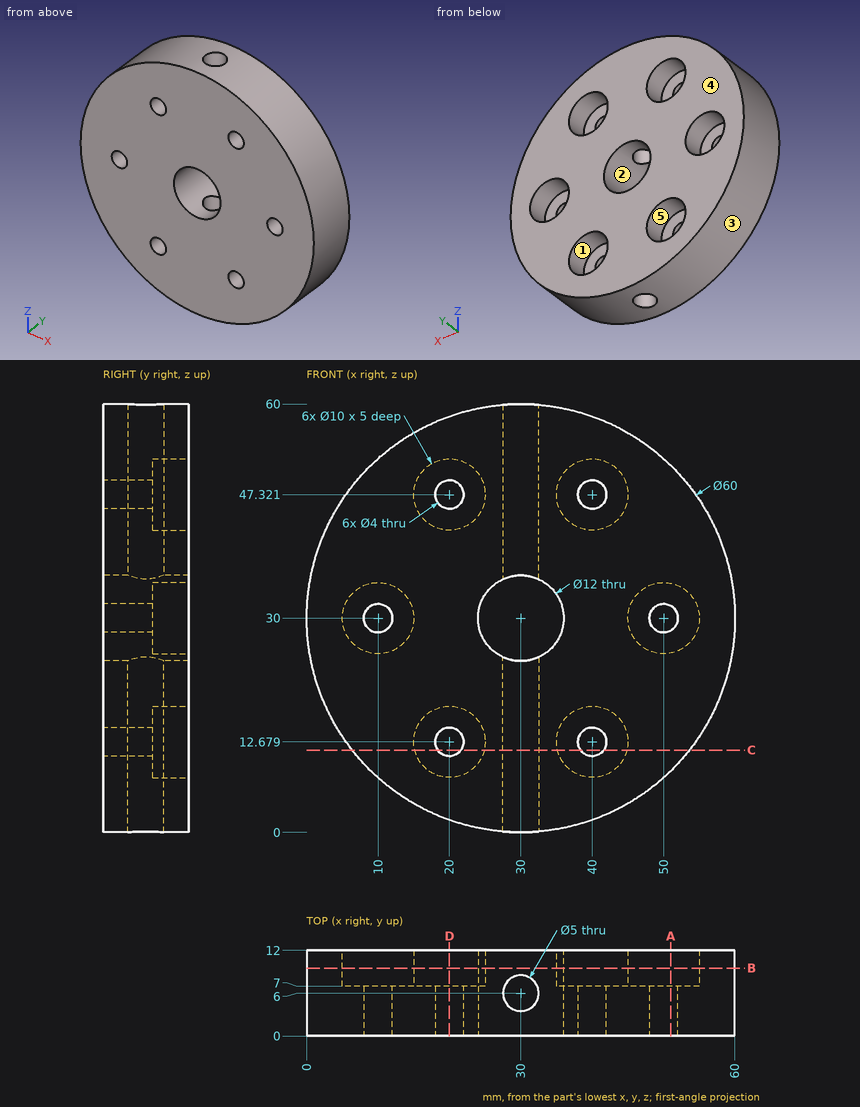
The drawing under review shows one solid part. Ordinate dimensions are in mm from its lowest x, y, z. A direction names the side the tool comes from. Coordinates: 2 decimals unless noted, no trailing zeros. Order: outer loops, then holes, each group sorted by start corner. A loop starts at its lowest first (then second) coordinate and runs counter-clockwise, first axis right, second up. Notation, with made-up numbers: (-29, 2) -> (21, 2) arc R23 cw to (21, 15) -> close; hole circle Ø7 at (55, 71). An arc over 180 degrees is marked (long way). Use CSV: the item, a comma, the result in double quotes. Start each with the question number.
Item 1: Draft analysis for pull direction Z (two halves, no side actions). For the marked faces 3, 4 and 5, state which applies: pulls with the +Z half, pulls with the -Z half, needs draft (parallel to the pull), parting line crosses it, or undercut.
Item 2: We need section C-C, the plane z = 11.5. Give the boundary of the cut face in (x, y) (1 decimal), then the cut area to 3 significant figures.
Item 3: Wall thickness on probe 1 along Z at (x, y) = (20, 5) (1 decimal); probe 2 along Y at (x, z) = (30, 52); probe 3 along X at (y, z) = (2.75, 46.5) (1 decimal): over which ranges is each line inside the solid? List them lowest first.
Item 4: We need section B-B, the plane y = 9.5. Give the boundary of the cut face in (x, z), then the cut area to 3 significant figures.
Item 5: We need section D-D, the plane x = 20. Give the boundary of the cut face in (y, z) (1 decimal).
Item 6: Insertion check: pin 1 (6 mm diameter, centred on x = 40, z = 12.68, fed in from +Y); pin 2 (3 mm diameter, centred on y = 5.5, z = 33.5, fed in from +X); pin 3 (1.5 mm diameter, centred on x = 36, y = 3, fed in from +Z). Each pin has a flat end and moves straight along its axis. Give the tip position at first contact, or say it passes through.
Item 7: For the marked faces 1 and 2, list the 3-axis set-ups (+Z, -Z, +X, -X, +Y, -Y) from which the entire face can be reached by the end or side of a thin tool; tool diameter is ignored.
Item 8: We need section A-A, the plane x = 51. Give the boundary of the cut face in (y, z) (1 decimal), then the cut area to 3 significant figures.
Derived:
1,face 3,"parting line crosses it"
1,face 4,"needs draft"
1,face 5,"undercut"
2,outline,"(6.4, 0) -> (18.4, 0) -> (18.4, 7) -> (15.1, 7) -> (15.1, 12) -> (6.4, 12) -> close; (21.6, 0) -> (38.4, 0) -> (38.4, 7) -> (35.1, 7) -> (35.1, 12) -> (24.9, 12) -> (24.9, 7) -> (21.6, 7) -> close; (41.6, 0) -> (53.6, 0) -> (53.6, 12) -> (44.9, 12) -> (44.9, 7) -> (41.6, 7) -> close; hole circle Ø5 at (30, 6)"
2,area,"405 mm^2"
3,probe 1,"z = 1.7 to 10.7, 14.7 to 45.3, 49.3 to 58.3"
3,probe 2,"y = 0 to 3.5, 8.5 to 12"
3,probe 3,"x = 4.9 to 18.2, 21.8 to 38.2, 41.8 to 55.1"
4,outline,"circle Ø60 at (30, 30); hole circle Ø10 at (10, 30); hole circle Ø10 at (20, 12.68); hole circle Ø10 at (20, 47.32); hole circle Ø12 at (30, 30); hole circle Ø10 at (40, 12.68); hole circle Ø10 at (40, 47.32); hole circle Ø10 at (50, 30)"
4,area,"2,240 mm^2"
5,outline,"(0, 1.7) -> (12, 1.7) -> (12, 7.7) -> (7, 7.7) -> (7, 10.7) -> (0, 10.7) -> close; (0, 14.7) -> (7, 14.7) -> (7, 17.7) -> (12, 17.7) -> (12, 42.3) -> (7, 42.3) -> (7, 45.3) -> (0, 45.3) -> close; (0, 49.3) -> (7, 49.3) -> (7, 52.3) -> (12, 52.3) -> (12, 58.3) -> (0, 58.3) -> close"
6,pin 1,"stops at y = 7"
6,pin 2,"stops at x = 59.93"
6,pin 3,"stops at z = 59.54"
7,face 1,"+Y"
7,face 2,"+Y, -Y"
8,outline,"(0, 8.6) -> (12, 8.6) -> (12, 25.1) -> (7, 25.1) -> (7, 28.3) -> (0, 28.3) -> close; (0, 31.7) -> (7, 31.7) -> (7, 34.9) -> (12, 34.9) -> (12, 51.4) -> (0, 51.4) -> close"
8,area,"441 mm^2"
